Autodesk Inventor part; units mm, degrees
ref_plane "YZ Plane" through (0, 0, 0) normal (1, 0, 0) x (0, 1, 0)
ref_plane "XZ Plane" through (0, 0, 0) normal (0, 1, 0) x (-1, 0, 0)
ref_plane "XY Plane" through (0, 0, 0) normal (0, 0, 1) x (1, 0, 0)
sketch "Sketch1" plane through (0, 0, 0) normal (0, 1, 0) x (-1, 0, 0)
  circle A0 centre (0, 0) radius 75
  circle A1 centre (0, 0) radius 85
  dimension "d1" = 150
  dimension "d2" = 170
extrude "Extrusion1" add sketch "Sketch1" along normal blind 250
sketch "Sketch2" plane through (0, 0, 0) normal (0, -1, 0) x (1, 0, 0)
  line L0 (-175, 250) -> (175, 250)
  line L1 (175, 250) -> (175, -250)
  line L2 (175, -250) -> (-175, -250)
  line L3 (-175, -250) -> (-175, 250)
  line L4 (-175, 250) -> (175, -250) construction
  line L5 (175, 250) -> (-175, -250) construction
  point P0 (0, 0)
  dimension "d5" = 500
  dimension "d6" = 350
extrude "Extrusion2" add sketch "Sketch2" along normal blind 500
sketch "Sketch3" plane through (0, -500, 0) normal (0, -1, 0) x (1, 0, 0)
  line L0 (-375, -375) -> (375, -375)
  line L1 (375, -375) -> (375, 375)
  line L2 (375, 375) -> (-375, 375)
  line L3 (-375, 375) -> (-375, -375)
  line L4 (-375, -375) -> (375, 375) construction
  line L5 (375, -375) -> (-375, 375) construction
  point P0 (0, 0)
  dimension "d9" = 750
  dimension "d10" = 750
extrude "Extrusion3" add sketch "Sketch3" along normal blind 100
fillet "Fillet2" radius 20 8 edges at (-175, -250, -250) (175, -250, -250) (-175, -250, 250) (175, -250, 250) (0, 0, 250) (175, 0, 0) (-175, 0, 0) (0, 0, -250)
fillet "Fillet3" radius 20 8 edges at (0, -600, -375) (0, -500, -375) (-375, -500, 0) (-375, -600, 0) (0, -600, 375) (0, -500, 375) (375, -500, 0) (375, -600, 0)
sketch "Sketch7" plane through (375, -520, -375) normal (0, 0, -1) x (-1, 0, 0)
  line L0 (750, 0) -> (0, 0)
  arc A0 (0, -60) -> (20, -80) centre (20, -60) ccw
  line L1 (0, 0) -> (0, -60)
  line L2 (109.0667, 0) -> (109.0667, -60)
  line L3 (1, -60) -> (749, -60)
  circle A1 centre (109.0667, -30) radius 22.5
  line L4 (375, 0) -> (375, -60)
  circle A2 centre (640.9333, -30) radius 22.5
  point P0 (375, 520)
  dimension "d27" = 45
extrude "Extrusion7" add sketch "Sketch7" along normal blind 90 contours A1 L2 | L2 A1 | A2
mirror "Mirror4" about plane through (0, 0, 0) normal (0, 0, 1) of "Extrusion7"
fillet "Fillet4" radius 10 4 edges at (-243.4333, -550, 465) (288.4333, -550, 465) (288.4333, -550, -465) (-243.4333, -550, -465)
properties part number "Base Prime" material "Aluminum 6061"
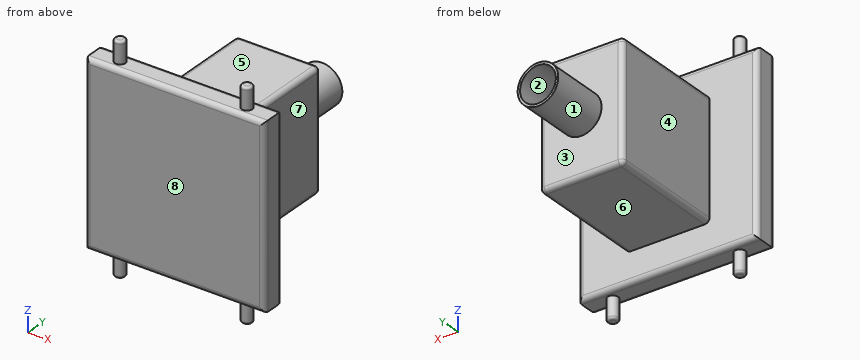
For this review, take the finished solid that the model builds, in its own axes (mm). Face numbers are marked on the shaded views. A direction names the side the tool comes from. Give positions to 0.01 mm unless a question says otherwise; leave off trailing zeros. Order: outer loops, then holes, each group sorted by start corner. A loop starts at its lowest first (then second) coordinate and runs counter-clockwise, first axis right, second up.
1) Take a section at D-D (y = 194). Give the boundary of the cut face in (x, z), then the cut area to 3 significant figures.
2) For the marked faces 5, 6, 7 and 8, list the 3-axis set-ups (+Z, -Z, +X, -X, +Y, -Y) from which the entire face can be reached by the end or side of a thin tool; tool diameter is ignored.
3) Wall thickness on line 1 (Z direction, x = 0, y = 155.5); line 2 (X direction, y = -441, z = 27.5); line 3 (Y direction, x = -18.5, z = 317.5): over which ranges is each line inside the solid? List them lowest first.
4) Take a section at B-B (x = 110). Give the boundary of the cut face in (y, z).
5) Insertion check: pin 1 (5 mm diameter, centred on y = -67.5, z = 226.5, fed in from -X); pin 2 (10 mm diameter, centred on y = -416, z = 207.5, fed in from +X); pin 3 (4 mm diameter, centred on x = -5.5, y = -415.5, fed in from +Z). Each pin has a flat end and moves straight along its axis. Give the tip position at first contact, or say it passes through.
6) Take a section at A-A (z = 0). Give the boundary of the cut face in (x, y), then the cut area to 3 significant figures.
7) The part is to be moulded in two halves that separate along X. For the marked faces 1, 2, 3 and 4, say which applies: released by +X, released by -X, zero draft, split by the parting line, or undercut.
8) Take a section at C-C (y = -42). Give the boundary of the cut face in (x, z).
Derived:
1. outline: circle Ø170 at (0, 0); hole circle Ø150 at (0, 0)
1. area: 5,030 mm2
2. face 5: +Z, +X, -X, +Y
2. face 6: -Z, +X, -X, +Y
2. face 7: +Z, -Z, +X, +Y
2. face 8: +Z, -Z, +X, -X, -Y
3. line 1: z = -85 to -75, 75 to 85
3. line 2: x = -175 to 175
3. line 3: y = -600 to -500
4. outline: (-600, -355) arc R20 ccw to (-580, -375) - (-520, -375) arc R20 ccw to (-500, -355) - (-500, -250) - (-20, -250) arc R20 ccw to (0, -230) - (0, 230) arc R20 ccw to (-20, 250) - (-500, 250) - (-500, 355) arc R20 ccw to (-520, 375) - (-580, 375) arc R20 ccw to (-600, 355) - close
5. pin 1: stops at x = -175
5. pin 2: stops at x = 175
5. pin 3: stops at z = 250
6. outline: (-375, -580) arc R20 ccw to (-355, -600) - (355, -600) arc R20 ccw to (375, -580) - (375, -520) arc R20 ccw to (355, -500) - (175, -500) - (175, -20) arc R20 ccw to (155, 0) - (85, 0) - (85, 250) - (75, 250) - (75, 0) - (-75, 0) - (-75, 250) - (-85, 250) - (-85, 0) - (-155, 0) arc R20 ccw to (-175, -20) - (-175, -500) - (-355, -500) arc R20 ccw to (-375, -520) - close
6. area: 254,000 mm2
7. face 1: split by the parting line
7. face 2: undercut
7. face 3: zero draft
7. face 4: released by -X
8. outline: (-175, -230) arc R20 ccw to (-155, -250) - (155, -250) arc R20 ccw to (175, -230) - (175, 230) arc R20 ccw to (155, 250) - (-155, 250) arc R20 ccw to (-175, 230) - close
